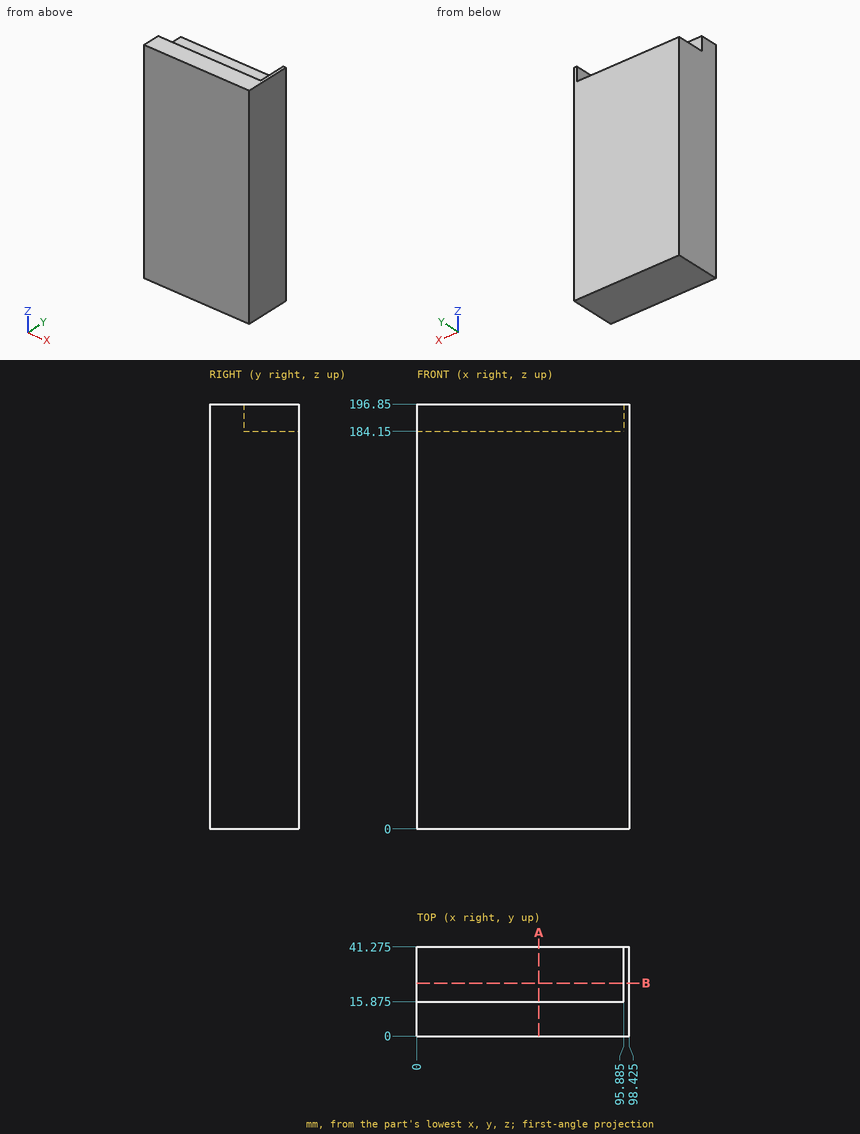
Drawing for the job (mm, zero at the part's lowest x, y, z). Give positions to 0.01 mm unless a question says otherwise; leave off trailing zeros. Write each loop counter-clockwise with the first axis right and the second up, starting at its lowest first coordinate (ties: lowest second). Pieces come first, ordered by that corner, then holes. Notation, with made-up numbers: M 4,-20 L 48,-20 A15 ccw 48,-9 Z; hole C 8.5,81 d6. An arc over 180 degrees is marked long. Return JSON: item names as keys, results as strings. Group by question number.
(1) Flat gauge pins, fed straight in: pin 1 Ø20.5 at (x, y) = (24.5, 34.5) entering from +Z; pin 2 Ø14 at (y, z) = (30, 193) entering from -X (3 decimals). Where does each tip first touch, or does it go through?
(2) Drill centre lines: L1, parallel to Z at x = 48, y = 39; L2, parallel to X at y = 38, z = 184.5 (3 decimals); L3, parallel to Y at x = 38, z = 186 (3 decimals). Where is each one in solid material? Low to high. Write a range as [from, to].
(3) Band-saw the part on A-A (x = 56.5). Give the cut face in (y, z) (3 decimals).
(4) Band-saw the part on B-B (y = 24.5). Give the cut face in (x, z) (3 decimals).
Entries:
{
 "1": {"pin 1": "stops at z = 184.15", "pin 2": "stops at x = 95.885"},
 "2": {"L1": "z = [0, 184.15]", "L2": "x = [95.885, 98.425]", "L3": "y = [0, 15.875]"},
 "3": {"outline": "M 0,0 L 41.275,0 L 41.275,184.15 L 15.875,184.15 L 15.875,196.85 L 0,196.85 Z"},
 "4": {"outline": "M 0,0 L 98.425,0 L 98.425,196.85 L 95.885,196.85 L 95.885,184.15 L 0,184.15 Z"}
}
